```python
from build123d import *

# Parameters (mm, degrees)
F1_DEPTH = 30
F2_W     = 3
F2_H     = 15
F3_DEPTH = 30
F2_W_2   = 4
F4_DEPTH = 30
F2_W_3   = 2
F2_H_2   = 7
F5_DEPTH = 30
F7_D     = 2.6416


with BuildPart() as f1:
    # F0 (on Right) → F1 (new body)
    with BuildSketch(Plane.YZ):
        Polygon((5.42, 14.5), (11, 8.92), (11, 20.08), align=None)
        Polygon((-11, 20.08), (-11, 8.92), (-5.42, 14.5), align=None)
        Polygon((-21, 4), (-21, 0), (0, 0), (0, 4), (-11, 4), align=None)
        Polygon((0, 4), (0, 0), (21, 0), (21, 4), (11, 4), align=None)
        Polygon((11, 4), (21, 4), (13, 25), (11, 25), (11, 20.08), (11, 8.92), align=None)
        Polygon((-13, 25), (-21, 4), (-11, 4), (-11, 8.92), (-11, 20.08), (-11, 25), align=None)
    extrude(amount=F1_DEPTH)

    # F2 (on Right) → F3 (join, through all)
    with BuildSketch(Plane.YZ):
        with Locations((-19.5, -7.5)):
            Rectangle(F2_W, F2_H)
        with Locations((9.5, -7.5)):
            Rectangle(F2_W, F2_H)
        with Locations((19.5, -7.5)):
            Rectangle(F2_W, F2_H)
    extrude(amount=F3_DEPTH)

    # F2 (on Right) → F4 (join, through all)
    with BuildSketch(Plane.YZ):
        with Locations((-9, -7.5)):
            Rectangle(F2_W_2, F2_H)
    extrude(amount=F4_DEPTH)

    # F2 (on Right) → F5 (join, through all)
    with BuildSketch(Plane.YZ):
        with Locations((-5, -3.5)):
            Rectangle(F2_W_3, F2_H_2)
    extrude(amount=F5_DEPTH)

    # F7 (through all)
    with Locations(Plane(origin=(0, 21, 0), x_dir=(-1, 0, 0), z_dir=(0, 1, 0))):
        with Locations((-15, -11)):
            Hole(F7_D / 2)


solid = f1.part
```
Geometry check sheet. Reference: the model listing, model coordinates, mm. A direction names the side the tool comes from. Round coordinates to 2 decimals unless told otherwise and drop trailing zeros. Write each loop counter-clockwise with the first axis right and the second up, starting at its lowest first coordinate (ties: lowest second). Pieces come first, ordered by that corner, then holes. Notation, with made-up numbers: (18.25, -4.75) -> (38.25, -4.75) arc R6 cw to (38.25, 3.25) -> close; hole circle Ø4 at (-7, 31.25). An arc over 180 degrees is marked (long way). Put each result on its own line as item: value.
1) Depth check by flat-ended pin: P1, Ø6, axis at x = 16.5, y = 0.5, coming from the -Z side; P2, Ø1.5, axis at x = 7.5, z = 21.5, coming from the +Y side; P3, Ø2.5, axis at x = 20.5, z = 6.5, coming from the -Y side; P4, Ø2.5, axis at x = 15, z = -11, coming from the -Y side (1 decimal). Enter the tip coordinate at first touch or a pass-through.
Recorded:
P1: stops at z = 0
P2: stops at y = 14.62
P3: stops at y = -20.52
P4: passes through
2) Thickness scan on probe 1 along Y at (x, z) = (1.75, -0.5); probe 2 along Z at (x, y) = (15, -9.9); probe 3 along Z at (x, y) = (15, 10). Record the ranges inside material, lowest first. Write a range as from..to.
Recorded:
probe 1: y = -21..-18, -11..-7, -6..-4, 8..11, 18..21
probe 2: z = -15..-12.32, -9.68..4, 10.02..18.98
probe 3: z = -15..-12.32, -9.68..4, 9.92..19.08
3) Cross-section at A-A, the plane z = -3. Enter the section's corners in (x, y), plus the area to 3 significant figures.
Recorded:
outline: (0, -21) -> (30, -21) -> (30, -18) -> (0, -18) -> close; (0, -11) -> (30, -11) -> (30, -7) -> (0, -7) -> close; (0, -6) -> (30, -6) -> (30, -4) -> (0, -4) -> close; (0, 8) -> (30, 8) -> (30, 11) -> (0, 11) -> close; (0, 18) -> (30, 18) -> (30, 21) -> (0, 21) -> close
area: 450 mm2
4) Cross-section at B-B, the plane z = -11. Give the number of separate pieces and of enclosed holes in the cut face, plus the area to 3 significant figures.
Recorded:
separate pieces: 8
enclosed holes: 0
area: 356 mm2
5) Access from +Z, -Z, +X, -X, +Y, -Y to the whole of each face (thin tool, end or side, straight path). Record for faces 1 (the face through (15, 0, 4)), 2 (the face through (15, -11, 23)), 3 (the face through (15, -18, -8)), 4 (the face through (15, -20, -15)).
Recorded:
face 1: +X, -X
face 2: +Z, +X, -X
face 3: -Z, +X, -X
face 4: -Z, +X, -X, +Y, -Y
6) Release check for a two-part mould opening along Y. For faces 5 (the face through (14.79, 17.056, 14.353)), 6 (the face through (15, -15, 0)), 7 (the face through (15, -9, -15)) record: pulls with the +Y half, pulls with the -Y half, needs draft (parallel to the pull), parting line crosses it, or undercut.
Recorded:
face 5: pulls with the +Y half
face 6: undercut
face 7: needs draft
